```python
from build123d import *


with BuildPart() as part:
    # Sketch1 → Revolve1 (revolve)
    with BuildSketch(Plane.XY):
        with BuildLine():
            Line((5.0165, 0), (9.280631004, 0))
            ThreePointArc((9.280631004, 0), (10.494721496, 0.308949961), (11.413463004, 1.160642302))
            ThreePointArc((11.413463004, 1.160642302), (12.040594592, 2.526079315), (12.2555, 4.0132))
            Line((12.2555, 4.0132), (10.7315, 4.0132))
            ThreePointArc((10.7315, 4.0132), (10.485243398, 2.680592322), (9.779, 1.524))
            Line((9.779, 1.524), (5.0165, 1.524))
            Line((5.0165, 1.524), (5.0165, 0))
        make_face()
    revolve(axis=Axis((0, 0, 0), (0, 1, 0)))


solid = part.part
```
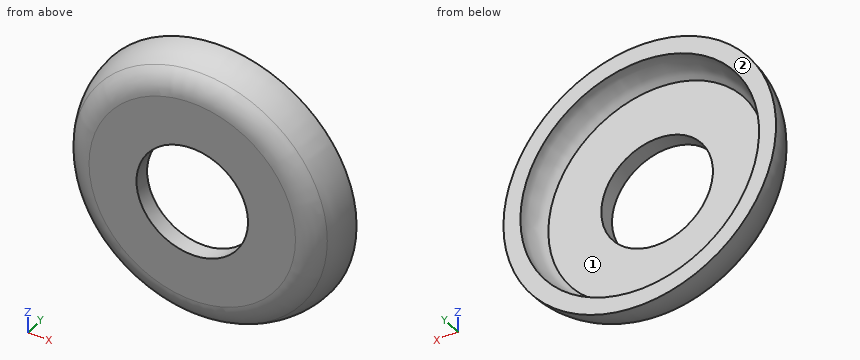
Could you check a few things on this model? Use its own coordinates, in mm. Face numbers are marked on the shaded views. Give positions to 0.01 mm unless a question says otherwise; leave off trailing zeros. Order: outer loops, then holes, each group sorted by start corner. A loop starts at its lowest first (then second) coordinate and runs counter-clockwise, first axis right, second up.
Q1. Suppose I cut it at D-D, the plane y = 2. Write out the boundary of the cut face in (x, z).
Q2. I'm going to push flat-ended pins straight in: P1, Ø1, axis at y = 0.5, z = 1, coming from the -X side; P2, Ø2, axis at x = 6.5, y = 2, coming from the -Z side. Where does each tip first touch, or does it pass through?
Q3. If I drill on line 1 along X through (y, z) = (1.15, 0); line 2 along Y through (x, z) = (-4.75, 3.5); line 3 along X through (y, z) = (0.65, 0), over which ranges is the centre line in solid material (lowest first)?
Q4. Suppose I cut it at C-C, the plane y = 3.3. Write out the boundary of the cut face in (x, z).
Q5. Suppose I cut it at A-A, the plane z = 0. Write out the boundary of the cut face in (x, y).
Q6. We'd pull the mould along X, two halves only. Please class the marked faces 1 and 2: +X half, -X half, draft (parallel to the pull), parting line (faces both ways), or undercut.
Q7. Suppose I cut it at B-B, the plane x = 0. Write out the boundary of the cut face in (y, z).
Solution:
1. outline: circle Ø23.71 at (0, 0); hole circle Ø20.28 at (0, 0)
2. P1: stops at x = -11.26
2. P2: stops at z = -10.63
3. line 1: x = -11.41 to -5.02, 5.02 to 11.41
3. line 2: y = 0 to 1.52
3. line 3: x = -10.98 to -5.02, 5.02 to 10.98
4. outline: circle Ø24.41 at (0, 0); hole circle Ø21.33 at (0, 0)
5. outline: (-12.26, 4.01) arc R5.25 ccw to (-11.41, 1.16) arc R2.54 ccw to (-9.28, 0) - (-5.02, 0) - (-5.02, 1.52) - (-9.78, 1.52) arc R3.73 cw to (-10.73, 4.01) - close; (5.02, 0) - (9.28, 0) arc R2.54 ccw to (11.41, 1.16) arc R5.25 ccw to (12.26, 4.01) - (10.73, 4.01) arc R3.73 cw to (9.78, 1.52) - (5.02, 1.52) - close
6. face 1: undercut
6. face 2: draft
7. outline: (0, -9.28) arc R2.54 ccw to (1.16, -11.41) arc R5.25 ccw to (4.01, -12.26) - (4.01, -10.73) arc R3.73 cw to (1.52, -9.78) - (1.52, -5.02) - (0, -5.02) - close; (0, 5.02) - (1.52, 5.02) - (1.52, 9.78) arc R3.73 cw to (4.01, 10.73) - (4.01, 12.26) arc R5.25 ccw to (1.16, 11.41) arc R2.54 ccw to (0, 9.28) - close
